Geometry check sheet. Reference: the model listing, model coordinates, mm. Face numbers are marked on the shaded views. A direction names the side the tool comes from. Coordinates: 2 decimals unless noted, no trailing zeros. Loops run counter-clockwise (first coordinate to the right, second up) from the corner with the lowest first, then second, coordinate; pieces in that order, holes last. Notation, with made-up numbers: (65, -14.75) - (115, -14.75) arc R23 cw to (115, 4.25) - close; hole circle Ø11 at (-14.75, 73). An arc over 180 degrees is marked (long way). One line per item, written item: value.
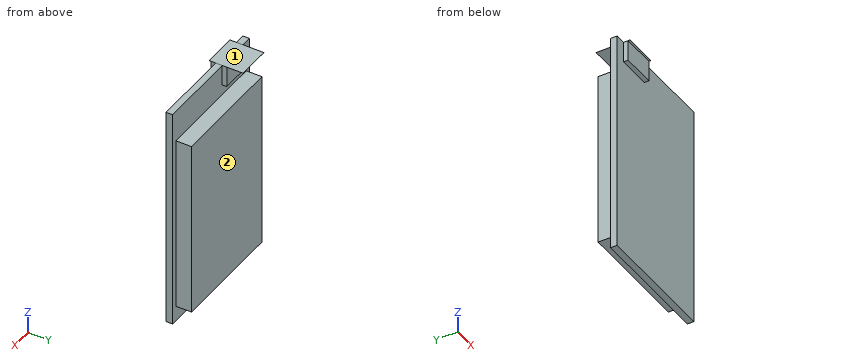
from build123d import *

# Parameters (mm, degrees)
SKETCH1_W               = 24
SKETCH1_H               = 43
PCB_DEPTH               = 1.25
SKETCH2_W               = 22
SKETCH2_H               = 34
RF_CASING_DEPTH         = 3
SKETCH3_W               = 6.5
SKETCH3_H               = 6.5
RF_CONNECTOR_BACK_DEPTH = 0.001
SKETCH5_W               = 6.5
SKETCH5_H               = 3
RF_CONNECTOR_PINS_DEPTH = 4


with BuildPart() as part:
    # Sketch1 → PCB (new body)
    with BuildSketch(Plane(origin=(0, 0, 0), x_dir=(1, 0, 0), z_dir=(0, 1, 0))):
        Rectangle(SKETCH1_W, SKETCH1_H)
    extrude(amount=PCB_DEPTH)

    # Sketch2 → RF Casing (add)
    with BuildSketch(Plane(origin=(0, 1.25, 0), x_dir=(1, 0, 0), z_dir=(0, 1, 0))):
        with Locations((0, 1.5)):
            Rectangle(SKETCH2_W, SKETCH2_H)
    extrude(amount=RF_CASING_DEPTH)

    # Sketch3 → RF Connector Back (add)
    with BuildSketch(Plane.XY.offset(21.5)):
        with Locations((-6.75, 2)):
            Rectangle(SKETCH3_W, SKETCH3_H)
    extrude(amount=RF_CONNECTOR_BACK_DEPTH)

    # Sketch5 → RF Connector Pins (add)
    with BuildSketch(Plane(origin=(0, 0, 21.5), x_dir=(-1, 0, 0), z_dir=(0, 0, -1))):
        with Locations((6.75, 0.625)):
            Rectangle(SKETCH5_W, SKETCH5_H)
    extrude(amount=RF_CONNECTOR_PINS_DEPTH)


solid = part.part
(1) Cross-section at B-B on z = 4. Record the cut outline in (x, y), and give its area (3 significant figures).
Reply:
outline: (-12, 0) - (12, 0) - (12, 1.25) - (11, 1.25) - (11, 4.25) - (-11, 4.25) - (-11, 1.25) - (-12, 1.25) - close
area: 96.0 mm2
(2) Material ranges on probe 1 along Z at (x, y) = (-8.5, 2); probe 2 along X at (y, z) = (2.25, 11.5); probe 3 along Y at (x, z) = (8.75, -2), recorded low to high. Write a range as from..to.
Reply:
probe 1: -18.5..15.5, 17.5..21.5
probe 2: -11..11
probe 3: 0..4.25
(3) Cross-section at D-D on z = 19.5. Record the cut outline in (x, y) (3 decimals).
Reply:
outline: (-12, 0) - (-10, 0) - (-10, -0.875) - (-3.5, -0.875) - (-3.5, 0) - (12, 0) - (12, 1.25) - (-3.5, 1.25) - (-3.5, 2.125) - (-10, 2.125) - (-10, 1.25) - (-12, 1.25) - close
(4) Go/stop test with flat-tipped pins: pin 1 Ø1.5 at (y, z) = (2.5, 6.5) entering from -X; pin 2 Ø6 at (x, z) = (-4, -4.5) entering from -Y; pin 3 Ø2 at (y, z) = (3, 19.5) entering from -X; pin 4 Ø0.7 at (x, y) = (-6.5, 1.5) entering from -Z. Record where each tip stops, or that it passes through.
Reply:
pin 1: x = -11
pin 2: y = 0
pin 3: x = -10
pin 4: z = -21.5
(5) Access from +Z, -Z, +X, -X, +Y, -Y to the whole of each face (thin tool, end or side, straight path). Record for the marked faces 1 and 2.
Reply:
face 1: +Z, +X, -X, +Y, -Y
face 2: -Z, +X, -X, +Y
